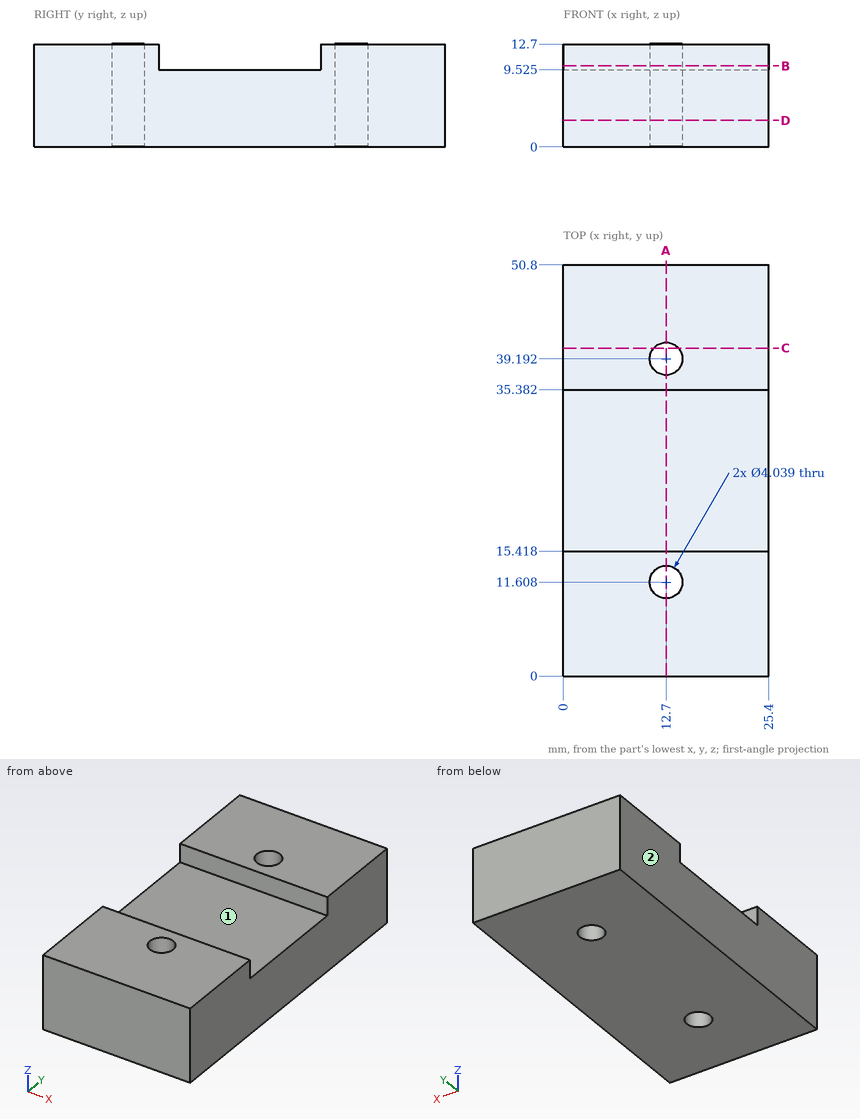
Print and shaded views of the part. All mm, measured from the part's lowest x, y and z. A direction names the side the tool comes from. Give positions to 0.01 mm unless a question says otherwise; leave off trailing zeros. Loops run counter-clockwise (first coordinate to the right, second up) from the corner with the lowest first, then second, coordinate; pieces in that order, holes last. Notation, with made-up numbers: (34.5, 50.5) -> (62.5, 50.5) arc R15 ccw to (62.5, 55.5) -> close; hole circle Ø5 at (-33, 33.5). An arc over 180 degrees is marked (long way). Use a Markdown table: item, result.
1. Which spindle directions (+Z, -Z, +X, -X, +Y, -Y) get a long thin tool onto all of the face, cutting with end or side? Do the marked faces 1 and 2. Say none if no direction does.
Check result:
| item | result |
|---|---|
| face 1 | +Z, +X, -X |
| face 2 | +Z, -Z, -X, +Y, -Y |
2. Flat gauge pin, fed straight in: pin 1 (5 mm diameter, centred on x = 18.5, z = 2.5, fed in from -Y). Where does the tip first touch, or does it go through?
Check result:
| item | result |
|---|---|
| pin 1 | stops at y = 0 |
3. Slice it at A-A (x = 12.7). List the corners of the cut face in (y, z) (1 decimal), plus the area to 3 significant figures.
Check result:
| item | result |
|---|---|
| outline | (0, 0) -> (9.6, 0) -> (9.6, 12.7) -> (0, 12.7) -> close; (13.6, 0) -> (37.2, 0) -> (37.2, 12.7) -> (35.4, 12.7) -> (35.4, 9.5) -> (15.4, 9.5) -> (15.4, 12.7) -> (13.6, 12.7) -> close; (41.2, 0) -> (50.8, 0) -> (50.8, 12.7) -> (41.2, 12.7) -> close |
| area | 479 mm^2 |
4. Slice it at B-B (z = 10). List the corners of the cut face in (x, y).
Check result:
| item | result |
|---|---|
| outline | (0, 0) -> (25.4, 0) -> (25.4, 15.42) -> (0, 15.42) -> close; (0, 35.38) -> (25.4, 35.38) -> (25.4, 50.8) -> (0, 50.8) -> close; hole circle Ø4.04 at (12.7, 11.61); hole circle Ø4.04 at (12.7, 39.19) |
5. Slice it at C-C (y = 40.5). List the corners of the cut face in (x, z).
Check result:
| item | result |
|---|---|
| outline | (0, 0) -> (11.16, 0) -> (11.16, 12.7) -> (0, 12.7) -> close; (14.24, 0) -> (25.4, 0) -> (25.4, 12.7) -> (14.24, 12.7) -> close |
6. Slice it at D-D (z = 3.25). List the corners of the cut face in (x, y).
Check result:
| item | result |
|---|---|
| outline | (0, 0) -> (25.4, 0) -> (25.4, 50.8) -> (0, 50.8) -> close; hole circle Ø4.04 at (12.7, 11.61); hole circle Ø4.04 at (12.7, 39.19) |
7. Wall check: L1, parallel to Y at x = 12.7, z = 8; L2, parallel to Y at x = 13.75, z = 10.75; L3, parallel to Z at x = 20.75, y = 30.5 (1 decimal). Give the ranges that are in metal, low to high. Write a range as [from, to].
Check result:
| item | result |
|---|---|
| L1 | y = [0, 9.59], [13.63, 37.17], [41.21, 50.8] |
| L2 | y = [0, 9.88], [13.33, 15.42], [35.38, 37.47], [40.92, 50.8] |
| L3 | z = [0, 9.5] |
